Read the model definition and answer for the solid it produces. Units are mm, in the model's axes. A direction names the side the tool comes from. Give positions to 0.01 mm unless a question says otherwise; leave off trailing zeros. Write each loop counter-clockwise with the first axis right and the second up, starting at its lowest first coordinate (ties: lowest second). Pieces come first, ordered by that corner, then holes.
```python
from build123d import *

# Parameters (mm, degrees)
F0_R     = 9.525
F1_DEPTH = 212.725
F2_R     = 7.9375
F3_DEPTH = 15.875
F3_TAPER = 3
F4_R     = 3.175
F5_DEPTH = 12.7


with BuildPart() as f1:
    # F0 (on Top) → F1 (new body)
    with BuildSketch(Plane.XY):
        Circle(F0_R)
    extrude(amount=-F1_DEPTH)

    # F2 (on face) → F3 (join)
    with BuildSketch(Plane.XY):
        Circle(F2_R)
    extrude(amount=F3_DEPTH, taper=F3_TAPER)

    # F4 (on Front) → F5 (cut, symmetric)
    with BuildSketch(Plane.XZ):
        with Locations((0, -200.025)):
            Circle(F4_R)
    extrude(amount=F5_DEPTH, both=True, mode=Mode.SUBTRACT)


solid = f1.part
```
Item 1: Which of the six approach directions +Z, -Z, +X, -X, +Y, -Y give full straight-line access (tool end or side, diameter ignored) to faces 4 (the flat face through (-2, 8, 0)), 5 (the cylindrical face through (9.085, 2.861, -104.873))?
Result set:
face 4: +Z
face 5: +Z, -Z
Item 2: Determine the mould class of faces 1 (the flat face through (0, 0, 15.875)), 2 (the flat face through (0, 0, -212.725)), 3 (the cylindrical face through (-0.688, -0.134, -203.124)) for opening direction Z: pulls with the +Z half, pulls with the -Z half, needs draft (parallel to the pull), parting line crosses it, or undercut.
Result set:
face 1: pulls with the +Z half
face 2: pulls with the -Z half
face 3: undercut
Item 3: Section C-C (z = -51) is taken. Write down the section's boundary in (x, y) (3 decimals), and give its area (3 significant figures).
Result set:
outline: circle Ø19.05 at (0, 0)
area: 285 mm2
Item 4: Find the intervals of material crossed by line 1 along Z through (x, y) = (0, 4) (3 decimals); line 2 along Z through (x, y) = (-5.5, -7) (3 decimals); line 3 along Y through (x, z) = (-0.75, -196), in increasing order.
Result set:
line 1: z = -212.725 to -203.2, -196.85 to 15.875
line 2: z = -212.725 to 0
line 3: y = -9.5 to 9.5
Item 5: Each of these flat-tipped pins is pushed along its axis until it touches: pin 1 Ø4 at (y, z) = (-1.5, -147) entering from -X (3 decimals); pin 2 Ø1 at (y, z) = (-3.5, -48.5) entering from +X; pin 3 Ø5 at (x, z) = (3.5, -174.5) entering from -Y; pin 4 Ø8 at (y, z) = (6.5, -172.5) entering from +X. Where does it stop, or does it pass through?
Result set:
pin 1: stops at x = -9.525
pin 2: stops at x = 9.04
pin 3: stops at y = -9.47
pin 4: stops at x = 9.19
